Autodesk Inventor part; units mm, degrees
ref_plane "YZ Plane" through (0, 0, 0) normal (1, 0, 0) x (0, 1, 0)
ref_plane "XZ Plane" through (0, 0, 0) normal (0, 1, 0) x (-1, 0, 0)
ref_plane "XY Plane" through (0, 0, 0) normal (0, 0, 1) x (1, 0, 0)
sketch "Sketch1" plane through (0, 0, 0) normal (0, 1, 0) x (-1, 0, 0)
  circle A0 centre (0, 0) radius 20
  circle A1 centre (0, 0) radius 15 construction
  circle A2 centre (0, -15) radius 1.75
  circle A3 centre (-15, 0) radius 1.75
  circle A4 centre (0, 15) radius 1.75
  circle A5 centre (15, 0) radius 1.75
  circle A6 centre (0, 0) radius 13.25
  point P0 (0, -13.25)
  point P1 (-13.25, 0)
  point P2 (0, 13.25)
  point P3 (13.25, 0)
  dimension "d0" = 40
  dimension "d1" = 30
  dimension "d2" = 3.5
  dimension "d3" = 3.5
  dimension "d4" = 3.5
  dimension "d5" = 3.5
extrude "Extrusion1" add sketch "Sketch1" along normal blind 3
sketch "Sketch2" plane through (0, 3, 0) normal (0, 1, 0) x (1, 0, 0)
  circle A0 centre (0, 0) radius 20
  circle A1 centre (0, 0) radius 23
  dimension "d8" = 46
extrude "Extrusion2" add sketch "Sketch2" against normal blind 30
properties part number "ColourSensor Scope"
Design review of the part built by this model. Coordinates are the model's own, in mm. A direction names the side the tool comes from. Round coordinates to 2 decimals unless told otherwise and drop trailing zeros. Order: outer loops, then holes, each group sorted by start corner. A loop starts at its lowest first (then second) coordinate and runs counter-clockwise, first axis right, second up. Notation, with made-up numbers: (45.5, 28) - (85.5, 28) arc R18 ccw to (85.5, 35) - close; hole circle Ø8 at (-37, 70.5). An arc over 180 degrees is marked (long way). One line per question, with ' | ' between items.
Item 1: Take a section at A-A, the plane z = 16. Write out the cut boundary in (x, y), then the cut area to 3 significant figures.
Checks:
outline: (-16.52, -27) - (-12, -27) - (-12, 0) - (-1.44, 0) - (-1.44, 3) - (-16.52, 3) - close; (1.44, 0) - (12, 0) - (12, -27) - (16.52, -27) - (16.52, 3) - (1.44, 3) - close | area: 335 mm²
Item 2: Wall thickness on line 1 (Z direction, x = 0.5, y = -4.5); line 2 (Y direction, x = 13, z = 3.5); line 3 (X direction, y = -12.25, z = 11.5): over which ranges is each line inside the solid? List them lowest first. Write a range as [from, to].
Checks:
line 1: [-22.99, -19.99], [19.99, 22.99] | line 2: [0, 3] | line 3: [-19.92, -16.36], [16.36, 19.92]
Item 3: For P1, Ø3, axis at y = -14, z = -6, coming from the -X side; P2, Ø1.5, axis at x = -17, z = 3, coming from the -Y side; P3, Ø1.5, axis at x = -13, y = -12, coming from the +Z side; P4, Ø4, axis at x = 0, z = 15, coming from the +Y side, all flat-tipped, find the tip position at first contact; note any pin that passes through.
Checks:
P1: x = -22.56 | P2: y = 0 | P3: z = 19.47 | P4: y = 3
Item 4: Take a section at B-B, the plane x = 16. Write out the cut boundary in (y, z), then the cut area to 3 significant figures.
Checks:
outline: (-27, -16.52) - (3, -16.52) - (3, -1.44) - (0, -1.44) - (0, -12) - (-27, -12) - close; (-27, 12) - (0, 12) - (0, 1.44) - (3, 1.44) - (3, 16.52) - (-27, 16.52) - close | area: 335 mm²
Item 5: Take a section at C-C, the plane y = -16.5. Write out the cut boundary in (x, z).
Checks:
outline: circle Ø46 at (0, 0); hole circle Ø40 at (0, 0)
Item 6: Draft analysis for pull direction Z (two halves, no side actions). For faces 4 (the face through (-10, 3, -10)), 5 (the face through (-13, 0, -4)), 6 (the face through (-2.994, -11.79, -22.804)), state which applies: +Z half, -Z half, draft (parallel to the pull), parting line (faces both ways), or undercut.
Checks:
face 4: draft | face 5: undercut | face 6: parting line
Item 7: Machinability: for faces 1 (the face through (-7, -27, -19)), 2 (the face through (-9.47, 1.48, -9.27)), 3 (the face through (-4.336, -13.311, 19.524)), which of the approach directions +Z, -Z, +X, -X, +Y, -Y give a long, thin tool a straight path to every point of the face, cutting with its end or side? Answer none if there is none.
Checks:
face 1: +Z, -Z, +X, -X, -Y | face 2: +Y, -Y | face 3: -Y
